```python
from build123d import *

# Parameters (mm, degrees)
ESQUISSE1_W             = 160
ESQUISSE1_H             = 210
BOSS_EXTRU_1_DEPTH      = 135
ESQUISSE2_W             = 265
ESQUISSE2_H             = 210
BOSS_EXTRU_2_DEPTH      = 5
ESQUISSE4_R             = 10
BOSS_EXTRU_3_DEPTH      = 60
BOSS_EXTRU_4_DEPTH      = 10
ESQUISSE6_W             = 154
ESQUISSE6_H             = 129
ENL_V_MAT_EXTRU_2_DEPTH = 30
ESQUISSE7_W             = 120
ESQUISSE7_H             = 140
ENL_V_MAT_EXTRU_3_DEPTH = 150
ESQUISSE9_R             = 5
ENL_V_MAT_EXTRU_4_DEPTH = 150


with BuildPart() as part:
    # Esquisse1 → Boss.-Extru.1 (new body)
    with BuildSketch(Plane.XY):
        Rectangle(ESQUISSE1_W, ESQUISSE1_H)
    extrude(amount=BOSS_EXTRU_1_DEPTH)

    # Esquisse2 → Boss.-Extru.2 (add)
    with BuildSketch(Plane.XY.offset(135)):
        Rectangle(ESQUISSE2_W, ESQUISSE2_H)
    extrude(amount=-BOSS_EXTRU_2_DEPTH)

    # Esquisse4 → Boss.-Extru.3 (add)
    with BuildSketch(Plane(origin=(80, 0, 0), x_dir=(0, 0, -1), z_dir=(1, 0, 0))):
        with Locations((-65, 0)):
            Circle(ESQUISSE4_R)
    boss_extru_3 = extrude(amount=BOSS_EXTRU_3_DEPTH)

    # Symétrie1: Boss.-Extru.3 across plane
    add(boss_extru_3.mirror(Plane(origin=(0, 0, 0), x_dir=(0, 0, 1), z_dir=(1, 0, 0))))

    # Esquisse5 → Boss.-Extru.4 (add)
    with BuildSketch(Plane(origin=(80, 0, 0), x_dir=(0, 0, -1), z_dir=(1, 0, 0))):
        with BuildLine():
            Line((-57.5, 30), (-48.218390917, 10.8801469))
            ThreePointArc((-48.218390917, 10.8801469), (-45.034127123, 1.167869962), (-47.064343322, -8.849419164))
            Line((-47.064343322, -8.849419164), (-57.5, -30))
            ThreePointArc((-57.5, -30), (-65, -37.5), (-72.5, -30))
            Line((-72.5, -30), (-82.935656678, -8.849419164))
            ThreePointArc((-82.935656678, -8.849419164), (-85, 0), (-82.935656678, 8.849419164))
            Line((-82.935656678, 8.849419164), (-72.5, 30))
            ThreePointArc((-72.5, 30), (-65, 37.5), (-57.5, 30))
        make_face()
    boss_extru_4 = extrude(amount=BOSS_EXTRU_4_DEPTH)

    # Symétrie2: Boss.-Extru.4 across plane
    add(boss_extru_4.mirror(Plane(origin=(0, 0, 0), x_dir=(0, 0, 1), z_dir=(1, 0, 0))))

    # Esquisse6 → Enlèv. mat.-Extru.2 (cut)
    with BuildSketch(Plane(origin=(0, 105, 0), x_dir=(1, 0, 0), z_dir=(0, 1, 0))):
        with Locations((0, -67.5)):
            Rectangle(ESQUISSE6_W, ESQUISSE6_H)
    enl_v_mat_extru_2 = extrude(amount=-ENL_V_MAT_EXTRU_2_DEPTH, mode=Mode.SUBTRACT)

    # Symétrie3: Enlèv. mat.-Extru.2 across plane
    add(enl_v_mat_extru_2.mirror(Plane.ZX), mode=Mode.SUBTRACT)

    # Esquisse7 → Enlèv. mat.-Extru.3 (cut)
    with BuildSketch(Plane(origin=(0, 0, 0), x_dir=(-1, 0, 0), z_dir=(0, 0, -1))):
        Rectangle(ESQUISSE7_W, ESQUISSE7_H)
    extrude(amount=-ENL_V_MAT_EXTRU_3_DEPTH, mode=Mode.SUBTRACT)

    # Esquisse9 → Enlèv. mat.-Extru.4 (cut)
    with BuildSketch(Plane(origin=(0, 0, 130), x_dir=(-1, 0, 0), z_dir=(0, 0, -1))):
        with Locations((-106.25, 80)):
            Circle(ESQUISSE9_R)
        with Locations((-106.25, -80)):
            Circle(ESQUISSE9_R)
    enl_v_mat_extru_4 = extrude(amount=-ENL_V_MAT_EXTRU_4_DEPTH, mode=Mode.SUBTRACT)

    # Symétrie4: Enlèv. mat.-Extru.4 across plane
    add(enl_v_mat_extru_4.mirror(Plane(origin=(0, 0, 0), x_dir=(0, 0, 1), z_dir=(1, 0, 0))), mode=Mode.SUBTRACT)


solid = part.part
```
The listing builds one solid part. Answer for the finished solid, in the listing's coordinates (mm). A direction names the side the tool comes from. Round coordinates to 2 decimals unless told otherwise and drop trailing zeros. Loops run counter-clockwise (first coordinate to the right, second up) from the corner with the lowest first, then second, coordinate; pieces in that order, holes last.
1) A cutting plane is placed at A-A on y = 80. Determine the outline of the cut face in (x, z), plus the area to 3 significant figures.
Outcome:
outline: (-132.5, 130) - (-111.25, 130) - (-111.25, 135) - (-132.5, 135) - close; (-101.25, 130) - (-80, 130) - (-80, 0) - (80, 0) - (80, 130) - (101.25, 130) - (101.25, 135) - (-101.25, 135) - close; (111.25, 130) - (132.5, 130) - (132.5, 135) - (111.25, 135) - close; hole (-77, 3) - (77, 3) - (77, 132) - (-77, 132) - close
area: 2,160 mm2
2) A cutting plane is placed at B-B on z = 124.5. Determine the outline of the cut face in (x, y), plus the area to 3 significant figures.
Outcome:
outline: (-80, -105) - (-77, -105) - (-77, -75) - (77, -75) - (77, -105) - (80, -105) - (80, 105) - (77, 105) - (77, 75) - (-77, 75) - (-77, 105) - (-80, 105) - close; hole (-60, -70) - (60, -70) - (60, 70) - (-60, 70) - close
area: 7,560 mm2
3) Given P1, Ø16, axis at x = 110, y = 46, coming from the -Z side; P2, Ø1.5, axis at x = -70.5, z = 21, coming from the -Y side; P3, Ø8, axis at y = -33.5, z = 68.5, coming from the -X side, each flat-ended and moving along its own axis, determine where each tip first touches the part or whether it passes through.
Outcome:
P1: stops at z = 130
P2: stops at y = -75
P3: stops at x = -90
4) A cutting plane is placed at C-C on x = -83.5. Determine the outline of the cut face in (y, z), plus the area to 3 significant figures.
Outcome:
outline: (-105, 130) - (105, 130) - (105, 135) - (-105, 135) - close; (-30, 57.5) - (-8.85, 47.06) arc R20 ccw to (10.88, 48.22) - (30, 57.5) arc R7.5 ccw to (30, 72.5) - (8.85, 82.94) arc R20 ccw to (-8.85, 82.94) - (-30, 72.5) arc R7.5 ccw to start
area: 2,990 mm2
5) For a pull along X with two mould halves and no side action, classify faces 1 (the face through (-1, -90, 132)), 2 (the face through (1, 70, 67)), 3 (the face through (-140, 0, 65)), 4 (the face through (84.93, -37.5, 64.84)) as released by +X, released by -X, zero draft, split by the parting line, or undercut.
Outcome:
face 1: undercut
face 2: undercut
face 3: released by -X
face 4: zero draft
6) Consider line 1 (Y direction, x = -106.25, z = 132.85); line 2 (X direction, y = -53.5, z = 6); line 3 (Y direction, x = 47, z = 107). Determine where each line is inside the solid, lowest interval first.
Outcome:
line 1: y = -105 to -85, -75 to 75, 85 to 105
line 2: x = -80 to -60, 60 to 80
line 3: y = -75 to -70, 70 to 75
7) For faces 5 (the face through (-84.93, 37.5, 65.16)), 6 (the face through (84.93, -19.28, 52.21)), 7 (the face through (-1, -90, 3)), 8 (the face through (84.93, 1.312, 45.043)), determine the directions among +Z, -Z, +X, -X, +Y, -Y from which every point of the face is accessible in a straight line to the end or side of a thin tool.
Outcome:
face 5: -X, +Y
face 6: -Z, +X, -Y
face 7: -Y
face 8: -Z, +X
8) A cutting plane is placed at D-D on y = 0. Determine the outline of the cut face in (x, z), plus the area to 4 significant figures.
Outcome:
outline: (-140, 55) - (-90, 55) - (-90, 45) - (-80, 45) - (-80, 0) - (-60, 0) - (-60, 135) - (-132.5, 135) - (-132.5, 130) - (-80, 130) - (-80, 85) - (-90, 85) - (-90, 75) - (-140, 75) - close; (60, 0) - (80, 0) - (80, 45) - (90, 45) - (90, 55) - (140, 55) - (140, 75) - (90, 75) - (90, 85) - (80, 85) - (80, 130) - (132.5, 130) - (132.5, 135) - (60, 135) - close
area: 8,725 mm2
